from build123d import *

# Parameters (mm, degrees)
SKETCH1_W           = 30.48
SKETCH1_H           = 24.13
BOSS_EXTRUDE1_DEPTH = 5.207
SKETCH2_W           = 24.13
SKETCH2_H           = 4.191
BOSS_EXTRUDE2_DEPTH = 5.842
FILLET5_START       = -22
FILLET5_DEPTH       = 37.24
FILLET5_START_2     = -13
FILLET5_2_DEPTH     = 26
FILLET4_R           = 0.381


with BuildPart() as part:
    # Sketch1 → Boss-Extrude1 (new body)
    with BuildSketch(Plane(origin=(0, 0, 0), x_dir=(1, 0, 0), z_dir=(0, 1, 0))):
        Rectangle(SKETCH1_W, SKETCH1_H)
    extrude(amount=BOSS_EXTRUDE1_DEPTH)

    # Sketch2 → Boss-Extrude2 (add)
    with BuildSketch(Plane.ZY.offset(15.24)):
        with Locations((0, 2.6035)):
            Rectangle(SKETCH2_W, SKETCH2_H)
    extrude(amount=BOSS_EXTRUDE2_DEPTH)

    # Fillet5: read off the stored shape, not the designer's step
    # Fillet5 outline → Fillet5 (cut)
    with BuildSketch(Plane.YZ.offset(FILLET5_START)):
        with BuildLine():
            Line((4.445, -12.065), (5.207, -12.065))
            Line((5.207, -12.065), (5.207, -11.303))
            ThreePointArc((5.207, -11.303), (4.983815367, -11.841815367), (4.445, -12.065))
        make_face()
        with BuildLine():
            ThreePointArc((0.762, -12.065), (0.223184633, -11.841815367), (0, -11.303))
            Line((0, -11.303), (0, -12.065))
            Line((0, -12.065), (0.762, -12.065))
        make_face()
        with BuildLine():
            Line((5.207, 12.065), (4.445, 12.065))
            ThreePointArc((4.445, 12.065), (4.983815367, 11.841815367), (5.207, 11.303))
            Line((5.207, 11.303), (5.207, 12.065))
        make_face()
        with BuildLine():
            Line((0.762, 12.065), (0, 12.065))
            Line((0, 12.065), (0, 11.303))
            ThreePointArc((0, 11.303), (0.223184633, 11.841815367), (0.762, 12.065))
        make_face()
    extrude(amount=FILLET5_DEPTH, mode=Mode.SUBTRACT)

    # Fillet5 2 outline → Fillet5 2 (cut)
    with BuildSketch(Plane.XY.offset(FILLET5_START_2)):
        with BuildLine():
            Line((-15.24, 5.207), (-15.24, 4.699))
            ThreePointArc((-15.24, 4.699), (-14.961520415, 5.067170395), (-14.52157951, 5.207))
            Line((-14.52157951, 5.207), (-15.24, 5.207))
        make_face()
        with BuildLine():
            Line((-15.24, 0), (-14.52157951, 0))
            ThreePointArc((-14.52157951, 0), (-14.961520415, 0.139829605), (-15.24, 0.508))
            Line((-15.24, 0.508), (-15.24, 0))
        make_face()
        with BuildLine():
            Line((15.24, 0), (15.24, 0.762))
            ThreePointArc((15.24, 0.762), (15.016815367, 0.223184633), (14.478, 0))
            Line((14.478, 0), (15.24, 0))
        make_face()
        with BuildLine():
            Line((15.24, 5.207), (14.478, 5.207))
            ThreePointArc((14.478, 5.207), (15.016815367, 4.983815367), (15.24, 4.445))
            Line((15.24, 4.445), (15.24, 5.207))
        make_face()
    extrude(amount=FILLET5_2_DEPTH, mode=Mode.SUBTRACT)

    # Fillet4
    # the kernel refuses this fillet: 0.381 mm, written as the material it takes off along each edge
    with BuildSketch(Plane(origin=(-21.082, 0.762, -12.065), x_dir=(1, 0, 0), z_dir=(0, 1, 0))) as fillet4_piece_1:
        with BuildLine():
            CenterArc((FILLET4_R, -FILLET4_R), FILLET4_R, 90, 90)
            Line((0, -FILLET4_R), (0, 0))
            Line((0, 0), (FILLET4_R, 0))
        make_face()
    extrude(amount=3.683, mode=Mode.SUBTRACT)
    with BuildSketch(Plane(origin=(-21.082, 4.445, 12.065), x_dir=(0, 0, -1), z_dir=(0, -1, 0))) as fillet4_piece_2:
        with BuildLine():
            CenterArc((FILLET4_R, FILLET4_R), FILLET4_R, 180, 90)
            Line((0, FILLET4_R), (0, 0))
            Line((0, 0), (FILLET4_R, 0))
        make_face()
    extrude(amount=3.683, mode=Mode.SUBTRACT)
    with BuildSketch(Plane(origin=(-21.082, 0.508, 12.973920489), x_dir=(0, 1, 0), z_dir=(0, 0, -1)), Plane(origin=(-21.082, 4.699, -12.973920489), x_dir=(0, -1, 0), z_dir=(0, 0, 1))) as fillet4_piece_3:
        with BuildLine():
            CenterArc((FILLET4_R, FILLET4_R), FILLET4_R, 180, 90)
            Line((0, FILLET4_R), (0, 0))
            Line((0, 0), (FILLET4_R, 0))
        make_face()
    extrude(amount=25.947840979, mode=Mode.SUBTRACT)
    with BuildSketch(Plane(origin=(-21.082, 4.444999999, 11.302999999), x_dir=(0, 1.1835443663887322e-09, 1.0), z_dir=(0, -1.0, 1.1835443663887322e-09))) as fillet4_piece_4:
        with BuildLine():
            CenterArc((0.762000001 - FILLET4_R, -FILLET4_R), FILLET4_R, 0, 90)
            Line((0.762000001, -FILLET4_R), (0.762000001, 0))
            Line((0.762000001, 0), (0.762000001 - FILLET4_R, 0))
        make_face()
    revolve(axis=Axis((-21.082, 4.444999999, 11.302999999), (-1, 0, 0)), revolution_arc=91.092291179, mode=Mode.SUBTRACT)
    with BuildSketch(Plane(origin=(-21.082, 0.762000001, 11.302999999), x_dir=(0, -0.9998182859562426, -0.019062923897481165), z_dir=(0, 0.019062923897481165, -0.9998182859562426))) as fillet4_piece_5:
        with BuildLine():
            CenterArc((0.762000001 - FILLET4_R, -FILLET4_R), FILLET4_R, 0, 90)
            Line((0.762000001, -FILLET4_R), (0.762000001, 0))
            Line((0.762000001, 0), (0.762000001 - FILLET4_R, 0))
        make_face()
    revolve(axis=Axis((-21.082, 0.762000001, 11.302999999), (-1, 0, 0)), revolution_arc=91.092291179, mode=Mode.SUBTRACT)
    with BuildSketch(Plane(origin=(-21.082, 0.762000001, -11.302999999), x_dir=(0, -1.1835437835944942e-09, -1.0), z_dir=(0, 1.0, -1.1835437835944942e-09))) as fillet4_piece_6:
        with BuildLine():
            CenterArc((0.762000001 - FILLET4_R, -FILLET4_R), FILLET4_R, 360, 90)
            Line((0.762000001, -FILLET4_R), (0.762000001, 0))
            Line((0.762000001, 0), (0.762000001 - FILLET4_R, 0))
        make_face()
    revolve(axis=Axis((-21.082, 0.762000001, -11.302999999), (-1, 0, 0)), revolution_arc=91.092291179, mode=Mode.SUBTRACT)
    with BuildSketch(Plane(origin=(-21.082, 4.444999999, -11.302999999), x_dir=(0, 0.9998182859562423, 0.019062923897497485), z_dir=(0, -0.019062923897497485, 0.9998182859562423))) as fillet4_piece_7:
        with BuildLine():
            CenterArc((0.762000001 - FILLET4_R, -FILLET4_R), FILLET4_R, 0, 90)
            Line((0.762000001 - FILLET4_R, 0), (0.762000001, 0))
            Line((0.762000001, 0), (0.762000001, -FILLET4_R))
        make_face()
    revolve(axis=Axis((-21.082, 4.444999999, -11.302999999), (-1, 0, 0)), revolution_arc=91.092291179, mode=Mode.SUBTRACT)


solid = part.part
Geometry: final body of the model. Coordinates: model frame, mm. A direction names the side the tool comes from. Give positions to 0.01 mm unless a question says otherwise; leave off trailing zeros. Order: outer loops, then holes, each group sorted by start corner. A loop starts at its lowest first (then second) coordinate and runs counter-clockwise, first axis right, second up. Notation, with made-up numbers: (-12.5, 19) -> (40.5, 19) arc R31 ccw to (40.5, 47) -> close; hole circle Ø7 at (-4, 6). An arc over 180 degrees is marked (long way). Put each result on its own line as item: value.
Q1. Section A-A, the plane x = -18. Return loops of the section in (y, z) (3 decimals), then the cut area to 3 significant figures.
Here are the results:
outline: (0.508, -12.021) arc R0.762 ccw to (0.762, -12.065) -> (4.445, -12.065) arc R0.762 ccw to (4.699, -12.021) -> (4.699, 12.021) arc R0.762 ccw to (4.445, 12.065) -> (0.762, 12.065) arc R0.762 ccw to (0.508, 12.021) -> close
area: 101 mm^2
Q2. Pin query (flat end, axial travel): pin 1 (1.6 mm diameter, centred on x = -17.5, z = 1, fed in from -Y); pin 2 (1.6 mm diameter, centred on x = -18, z = 3, fed in from +Y). Return the tip coordinate at first contact, or that it passes through.
Here are the results:
pin 1: stops at y = 0.51
pin 2: stops at y = 4.7
Q3. Reachability of faces 1 (the face through (0, 0, 0)), 2 (the face through (-18, 4.699, 0)), 3 (the face through (-18, 0.508, 0)) from +Z, -Z, +X, -X, +Y, -Y: full face, straight path, thin tool, end or side. Return the list, or none.
Here are the results:
face 1: +Z, -Z, +X, -X, -Y
face 2: +Z, -Z, -X, +Y
face 3: +Z, -Z, -X, -Y
Q4. Material intervals for L1, parallel to Y at x = -16, z = -3; L2, parallel to Z at x = 2.5, y = 4.55; L3, parallel to X at y = 0.75, z = -1.75, sorted ascending.
Here are the results:
L1: y = 0.51 to 4.7
L2: z = -12.06 to 12.06
L3: x = -21.06 to 15.24
Q5. Section B-B, the plane z = -10.25. Return loops of the section in (x, y) (3 decimals).
Here are the results:
outline: (-21.082, 0.889) arc R0.381 ccw to (-20.701, 0.508) -> (-15.24, 0.508) arc R0.762 ccw to (-14.522, 0) -> (14.478, 0) arc R0.762 ccw to (15.24, 0.762) -> (15.24, 4.445) arc R0.762 ccw to (14.478, 5.207) -> (-14.522, 5.207) arc R0.762 ccw to (-15.24, 4.699) -> (-20.701, 4.699) arc R0.381 ccw to (-21.082, 4.318) -> close
